Design review of the part built by this model. Coordinates are the model's own, in mm. Coordinates: 2 decimals unless noted, no trailing zeros. Loops run counter-clockwise (first coordinate to the right, second up) from the corner with the lowest first, then second, coordinate; pieces in that order, holes last. Notation, with made-up numbers: M 65.25,74 L 113.25,74 A19 ccw 113.25,90 Z; hole C 35,14 d9. An arc over 180 degrees is marked long. Answer as a JSON object with one key per item and string values. Group by question number.
1. Insertion check: pin 1 (6 mm diameter, centred on y = -25.5, z = 745, fed in from -X); pin 2 (4 mm diameter, centred on x = -0.5, z = 437, fed in from -Y); pin 3 (1 mm diameter, centred on y = 27.5, z = 593.5, fed in from -X). Each pin has a flat end and moves straight along its axis. Give the tip position at first contact, or say it passes through.
2. To check wall thickness, follow probe 1 along Y at (x, z) = (123.5, 311.5); probe 2 along Y at (x, z) = (150, 895); probe 3 along X at (y, z) = (86.5, 284). State the ranges of each line that lie inside material, in increasing order.
3. Consider section C-C (x = -87). State the section outline as (y, z) points, then the cut area to 3 significant figures.
4. Consider section B-B (y = 140). State the section outline as (x, z) points, then the cut area to 3 significant figures.
5. Consider section D-D (y = -66). State the section outline as (x, z) points.
6. Consider section A-A (z = 224). State the section outline as (x, y) points, then the cut area to 3 significant figures.
7. Draft analysis for pull direction X (two halves, no side actions). For faces 1 (the flat face through (-2, 2, 1060)), 2 (the cylindrical face through (-86.9, 151.9, 522.6)), 3 (the cylindrical face through (-0.91, -130.01, 522.58)), 4 (the cylindrical face through (113.045, 64.218, 522.58)), state which applies: +X half, -X half, draft (parallel to the pull), parting line (faces both ways), or undercut.
from build123d import *

# Parameters (mm, degrees)
F1_DEPTH = 1060


with BuildPart() as f1:
    # F0 (on Top) → F1 (new body)
    with BuildSketch(Plane.XY):
        with BuildLine():
            ThreePointArc((168.857126, -45.95945), (173.457483, -23.184079), (175, 0))
            ThreePointArc((175, 0), (173.457483, 23.184079), (168.857126, 45.95945))
            ThreePointArc((168.857126, 45.95945), (112.583302, 65), (124.230614, 123.254835))
            ThreePointArc((124.230614, 123.254835), (87.5, 151.554446), (44.626511, 169.214286))
            ThreePointArc((44.626511, 169.214286), (0, 130), (-44.626511, 169.214286))
            ThreePointArc((-44.626511, 169.214286), (-87.5, 151.554446), (-124.230614, 123.254835))
            ThreePointArc((-124.230614, 123.254835), (-111.21481, 107.442763), (-106.554446, 87.5))
            ThreePointArc((-106.554446, 87.5), (-126.590678, 50.059243), (-168.857126, 45.95945))
            ThreePointArc((-168.857126, 45.95945), (-175, 0), (-168.857126, -45.95945))
            ThreePointArc((-168.857126, -45.95945), (-126.590678, -50.059243), (-106.554446, -87.5))
            ThreePointArc((-106.554446, -87.5), (-111.21481, -107.442763), (-124.230614, -123.254835))
            ThreePointArc((-124.230614, -123.254835), (-87.5, -151.554446), (-44.626511, -169.214286))
            ThreePointArc((-44.626511, -169.214286), (0, -130), (44.626511, -169.214286))
            ThreePointArc((44.626511, -169.214286), (87.5, -151.554446), (124.230614, -123.254835))
            ThreePointArc((124.230614, -123.254835), (112.583302, -65), (168.857126, -45.95945))
        make_face()
    extrude(amount=F1_DEPTH)


solid = f1.part
Findings below:
{
 "1": {"pin 1": "stops at x = -173.55", "pin 2": "stops at y = -130.07", "pin 3": "stops at x = -172.9"},
 "2": {"probe 1": "y = -123.99 to -122.68, -52.32 to 52.32, 122.68 to 123.99", "probe 2": "y = -42.53 to 42.53", "probe 3": "x = -106.57 to 106.57"},
 "3": {"outline": "M -151.84,0 L 151.84,0 L 151.84,1060 L -151.84,1060 Z", "area": "322,000 mm^2"},
 "4": {"outline": "M -105,0 L -28.28,0 L -28.28,1060 L -105,1060 Z; M 28.28,0 L 105,0 L 105,1060 L 28.28,1060 Z", "area": "163,000 mm^2"},
 "5": {"outline": "M -112.02,0 L 112.02,0 L 112.02,1060 L -112.02,1060 Z"},
 "6": {"outline": "M -168.86,-45.96 A45 cw -106.55,-87.5 A45 cw -124.23,-123.25 A175 ccw -44.63,-169.21 A45 cw 44.63,-169.21 A175 ccw 124.23,-123.25 A45 cw 168.86,-45.96 A175 ccw 175,0 A175 ccw 168.86,45.96 A45 cw 124.23,123.25 A175 ccw 44.63,169.21 A45 cw -44.63,169.21 A175 ccw -124.23,123.25 A45 cw -106.55,87.5 A45 cw -168.86,45.96 A175 ccw Z", "area": "78,200 mm^2"},
 "7": {"face 1": "draft", "face 2": "-X half", "face 3": "undercut", "face 4": "undercut"}
}
